```python
from build123d import *

# Parameters (mm, degrees)
SKETCH1_R           = 18
BOSS_EXTRUDE1_DEPTH = 25
CUT_EXTRUDE1_DEPTH  = 10
FILLET1_R           = 10


with BuildPart() as part:
    # Sketch1 → Boss-Extrude1 (new body)
    with BuildSketch(Plane.XY):
        with BuildLine():
            Line((-21.031401564, -6.456016438), (-13.695019248, -30.355336397))
            Line((-13.695019248, -30.355336397), (13.695019248, -30.355336397))
            Line((13.695019248, -30.355336397), (21.031401564, -6.456016438))
            ThreePointArc((21.031401564, -6.456016438), (0, 22), (-21.031401564, -6.456016438))
        make_face()
        Circle(SKETCH1_R, mode=Mode.SUBTRACT)
    extrude(amount=BOSS_EXTRUDE1_DEPTH)

    # Sketch2 → Cut-Extrude1 (cut)
    with BuildSketch(Plane.XZ.offset(30.355336397)):
        with BuildLine():
            Line((-7, 12.5), (-4.5, 12.5))
            Line((-4.5, 12.5), (-2, 12.5))
            ThreePointArc((-2, 12.5), (-4.5, 15), (-7, 12.5))
        make_face()
        with BuildLine():
            Line((-2, 12.5), (-4.5, 12.5))
            Line((-4.5, 12.5), (-7, 12.5))
            ThreePointArc((-7, 12.5), (-4.5, 10), (-2, 12.5))
        make_face()
        with BuildLine():
            ThreePointArc((7, 12.5), (4.5, 15), (2, 12.5))
            Line((2, 12.5), (4.5, 12.5))
            Line((4.5, 12.5), (7, 12.5))
        make_face()
        with BuildLine():
            Line((4.5, 12.5), (2, 12.5))
            ThreePointArc((2, 12.5), (4.5, 10), (7, 12.5))
            Line((7, 12.5), (4.5, 12.5))
        make_face()
    extrude(amount=-CUT_EXTRUDE1_DEPTH, mode=Mode.SUBTRACT)

    # Fillet1
    fillet1_edges = [part.edges().sort_by_distance(p)[0] for p in [
        (0, -30.355336397, 25),
        (0, -30.355336397, 0),
    ]]
    fillet(fillet1_edges, radius=FILLET1_R - 0.0001)  # a hair under: the kernel refuses the full size


solid = part.part
```
Source: CAD feature listing. Evaluate the final solid. Frame: model axes, mm. A direction names the side the tool comes from. Give positions to 0.01 mm unless a question says otherwise; leave off trailing zeros. Loops run counter-clockwise (first coordinate to the right, second up) from the corner with the lowest first, then second, coordinate; pieces in that order, holes last. Notation, with made-up numbers: (61, 33.25) - (114, 33.25) arc R24 cw to (114, 49.25) - close; hole circle Ø3 at (66.5, 13). An arc over 180 degrees is marked (long way). Use CSV: the item, a comma, the result in double quotes. Start each with the question number.
1. Section C-C (z = 12.5). Output: boundary loops of the cut face in (x, y).
2. Section A-A (x = -13). Output: boundary loops of the cut face in (y, z), then the cut area to 3 significant figures.
3. Draft query along Z for faces 3 (the cylindrical face through (0.575, 21.992, 12.325)), 4 (the flat face through (-3, -18, 0)), 5 (the flat face through (-5, -20.355, 13)), 6 (the cylindrical face through (3.35, -25.43, 14.72)). Return one class per face: +Z half, -Z half, draft (parallel to the pull), parting line (faces both ways), or undercut.
4. Ray query, L1, parallel to X at y = -25.5, z = 12.5; L2, parallel to X at y = -25.25, z = 12.5; L3, parallel to Y at x = 0, z = 13. Return the intervals inside material, ascending.
5. Section B-B (y = 4). Output: boundary loops of the cut face in (x, z).
6. Pin query (flat end, axial travel): pin 1 (2.5 mm diameter, centred on x = 5, z = 13, fed in from -Y); pin 2 (4.5 mm diameter, centred on x = 4.5, z = 12.5, fed in from +Y); pin 3 (12 mm diameter, centred on y = -16, z = 5.5, fed in from +X). Return the tip coordinate at first contact, or that it passes through.
7. Reachability of faces 1 (the flat face through (4, -20.355, 13)), 2 (the flat face through (-3, -18, 25)) from +Z, -Z, +X, -X, +Y, -Y: full face, straight path, thin tool, end or side. Return the list, or none.
8. Section D-D (x = 0). Output: boundary loops of the cut face in (y, z).
Response:
1,outline,"(-21.03, -6.46) - (-13.7, -30.36) - (-7, -30.36) - (-7, -20.36) - (-2, -20.36) - (-2, -30.36) - (2, -30.36) - (2, -20.36) - (7, -20.36) - (7, -30.36) - (13.7, -30.36) - (21.03, -6.46) arc R22 ccw (long way) to start; hole circle Ø36 at (0, 0)"
2,outline,"(-30.36, 10) arc R10 ccw to (-20.36, 0) - (-12.45, 0) - (-12.45, 25) - (-20.36, 25) arc R10 ccw to (-30.36, 15) - close; (12.45, 0) - (17.75, 0) - (17.75, 25) - (12.45, 25) - close"
2,area,"537 mm²"
3,face 3,"draft"
3,face 4,"-Z half"
3,face 5,"undercut"
3,face 6,"undercut"
4,L1,"-15.19 to -7, -2 to 2, 7 to 15.19"
4,L2,"-15.26 to -7, -2 to 2, 7 to 15.26"
4,L3,"-30.36 to -18, 18 to 22"
5,outline,"(-21.63, 0) - (-17.55, 0) - (-17.55, 25) - (-21.63, 25) - close; (17.55, 0) - (21.63, 0) - (21.63, 25) - (17.55, 25) - close"
6,pin 1,"y = -20.36"
6,pin 2,"y = 21.88"
6,pin 3,"x = 19.94"
7,face 1,"-Y"
7,face 2,"+Z, +X, -X, +Y, -Y"
8,outline,"(-30.36, 10) arc R10 ccw to (-20.36, 0) - (-18, 0) - (-18, 25) - (-20.36, 25) arc R10 ccw to (-30.36, 15) - close; (18, 0) - (22, 0) - (22, 25) - (18, 25) - close"
